Check sheet for the modelled part. Datum: model origin and axes. Units: mm. Coordinates: 2 decimals unless noted, no trailing zeros. Order: outer loops, then holes, each group sorted by start corner. A loop starts at its lowest first (then second) coordinate and runs counter-clockwise, first axis right, second up. Notation, with made-up numbers: M 85.25,75 L 114.25,75 A27 cw 114.25,95 Z; hole C 33.25,-2.5 d3. An arc over 180 degrees is marked long. Answer in a Markdown table with one row per item. Add a question column.
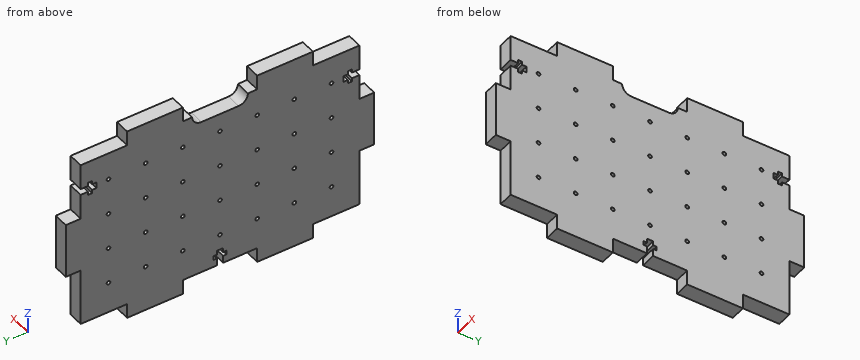
from build123d import *

# Parameters (mm, degrees)
SKETCH1_W           = 92
SKETCH1_H           = 150
BOSS_EXTRUDE1_DEPTH = 8
SKETCH2_W           = 30
SKETCH2_H           = 8
SKETCH2_W_2         = 8
SKETCH2_H_2         = 30
BOSS_EXTRUDE2_DEPTH = 8
SKETCH3_R           = 1
CUT_EXTRUDE1_DEPTH  = 8
CUT_EXTRUDE2_DEPTH  = 9
CUT_EXTRUDE4_DEPTH  = 9


with BuildPart() as part:
    # Sketch1 → Boss-Extrude1 (new body)
    with BuildSketch(Plane(origin=(0, 0, 0), x_dir=(0, 0, -1), z_dir=(1, 0, 0))):
        with Locations((46, 75)):
            Rectangle(SKETCH1_W, SKETCH1_H)
    extrude(amount=BOSS_EXTRUDE1_DEPTH)

    # Sketch2 → Boss-Extrude2 (add)
    with BuildSketch(Plane.ZY):
        with Locations((-46, 154)):
            Rectangle(SKETCH2_W, SKETCH2_H)
        with Locations((-46, -4)):
            Rectangle(SKETCH2_W, SKETCH2_H)
        with Locations((4, 40)):
            Rectangle(SKETCH2_W_2, SKETCH2_H_2)
        with Locations((4, 110)):
            Rectangle(SKETCH2_W_2, SKETCH2_H_2)
        with Locations((-96, 40)):
            Rectangle(SKETCH2_W_2, SKETCH2_H_2)
        with Locations((-96, 110)):
            Rectangle(SKETCH2_W_2, SKETCH2_H_2)
    extrude(amount=-BOSS_EXTRUDE2_DEPTH)

    # Sketch3 → Cut-Extrude1 (cut)
    with BuildSketch(Plane(origin=(8, 0, 0), x_dir=(0, 0, -1), z_dir=(1, 0, 0))):
        with Locations((15, 135)):
            Circle(SKETCH3_R)
        with Locations((35, 135)):
            Circle(SKETCH3_R)
        with Locations((55, 135)):
            Circle(SKETCH3_R)
        with Locations((75, 135)):
            Circle(SKETCH3_R)
        with Locations((15, 115)):
            Circle(SKETCH3_R)
        with Locations((35, 115)):
            Circle(SKETCH3_R)
        with Locations((55, 115)):
            Circle(SKETCH3_R)
        with Locations((75, 115)):
            Circle(SKETCH3_R)
        with Locations((15, 95)):
            Circle(SKETCH3_R)
        with Locations((35, 95)):
            Circle(SKETCH3_R)
        with Locations((55, 95)):
            Circle(SKETCH3_R)
        with Locations((75, 95)):
            Circle(SKETCH3_R)
        with Locations((15, 75)):
            Circle(SKETCH3_R)
        with Locations((35, 75)):
            Circle(SKETCH3_R)
        with Locations((55, 75)):
            Circle(SKETCH3_R)
        with Locations((75, 75)):
            Circle(SKETCH3_R)
        with Locations((15, 55)):
            Circle(SKETCH3_R)
        with Locations((35, 55)):
            Circle(SKETCH3_R)
        with Locations((55, 55)):
            Circle(SKETCH3_R)
        with Locations((75, 55)):
            Circle(SKETCH3_R)
        with Locations((15, 35)):
            Circle(SKETCH3_R)
        with Locations((35, 35)):
            Circle(SKETCH3_R)
        with Locations((55, 35)):
            Circle(SKETCH3_R)
        with Locations((75, 35)):
            Circle(SKETCH3_R)
        with Locations((15, 15)):
            Circle(SKETCH3_R)
        with Locations((35, 15)):
            Circle(SKETCH3_R)
        with Locations((55, 15)):
            Circle(SKETCH3_R)
        with Locations((75, 15)):
            Circle(SKETCH3_R)
    extrude(amount=-CUT_EXTRUDE1_DEPTH, mode=Mode.SUBTRACT)

    # Sketch4 → Cut-Extrude2 (cut, through all)
    with BuildSketch(Plane(origin=(8, 0, 0), x_dir=(0, 0, -1), z_dir=(1, 0, 0))):
        with BuildLine():
            Line((5, 85), (5, 65))
            ThreePointArc((5, 65), (0, 60), (-5, 65))
            Line((-5, 65), (-5, 85))
            ThreePointArc((-5, 85), (0, 90), (5, 85))
        make_face()
    extrude(amount=-CUT_EXTRUDE2_DEPTH, mode=Mode.SUBTRACT)

    # Sketch5 → Cut-Extrude4 (cut, through all)
    with BuildSketch(Plane(origin=(8, 0, 0), x_dir=(0, 0, -1), z_dir=(1, 0, 0))):
        Polygon((92, 76.65), (88, 76.65), (88, 78.5), (85.8, 78.5), (85.8, 76.65), (83.5, 76.65), (83.5, 73.35), (85.8, 73.35), (85.8, 71.5), (88, 71.5), (88, 73.35), (92, 73.35), align=None)
        Polygon((17.15, 0), (17.15, 4), (19, 4), (19, 6.2), (17.15, 6.2), (17.15, 8.5), (13.85, 8.5), (13.85, 6.2), (12, 6.2), (12, 4), (13.85, 4), (13.85, 0), align=None)
        Polygon((13.85, 150), (17.15, 150), (17.15, 146), (19, 146), (19, 143.8), (17.15, 143.8), (17.15, 141.5), (13.85, 141.5), (13.85, 143.8), (12, 143.8), (12, 146), (13.85, 146), align=None)
    extrude(amount=-CUT_EXTRUDE4_DEPTH, mode=Mode.SUBTRACT)


solid = part.part
1. Section check A-A on z = -78. Enter the section's corners in (x, y), then the cut area to 3 significant figures.
2. Scan lines: line 1 (Y direction, x = 7.25, z = -13); line 2 (Z direction, x = 1.5, y = 78); line 3 (Z direction, x = 6, y = 135). Record each from-to range of solid material in increasing order.
3. Go/stop test with flat-tipped pins: pin 1 Ø2 at (x, z) = (2.5, -13) entering from +Y; pin 2 Ø1 at (x, y) = (7, 83.5) entering from +Z; pin 3 Ø1.5 at (x, y) = (4.5, 126.5) entering from -Z; pin 4 Ø1.2 at (y, z) = (135, -55) entering from -X. Record where each tip stops, or that it passes through.
4. Section check B-B on x = 3.75. State how many separate pieces and enclosed holes the cut face has, then the cut area to 3 significant figures.
Result sheet:
| question | item | result |
|---|---|---|
| 1 | outline | M 0,0 L 8,0 L 8,150 L 0,150 Z |
| 1 | area | 1,200 mm^2 |
| 2 | line 1 | 0 to 4, 6.2 to 143.8, 146 to 150 |
| 2 | line 2 | -92 to -88, -85.8 to -5 |
| 2 | line 3 | -92 to -76, -74 to -56, -54 to -36, -34 to -16, -14 to 0 |
| 3 | pin 1 | y = 150 |
| 3 | pin 2 | z = -5 |
| 3 | pin 3 | z = -92 |
| 3 | pin 4 | through |
| 4 | separate pieces | 1 |
| 4 | enclosed holes | 28 |
| 4 | area | 14,900 mm^2 |
